```python
from build123d import *

# Parameters (mm, degrees)
F1_DEPTH = 20
F3_R     = 2
F5_DEPTH = 25
F6_R     = 2


with BuildPart() as f1:
    # F0 (on Front) → F1 (new body)
    with BuildSketch(Plane.XZ):
        with BuildLine():
            Line((-230, -180), (250, -180))
            ThreePointArc((250, -180), (264.142136, -174.142136), (270, -160))
            Line((270, -160), (270, -20))
            ThreePointArc((270, -20), (258.284271, 8.284271), (230, 20))
            Line((230, 20), (200, 20))
            Line((200, 20), (200, 140))
            ThreePointArc((200, 140), (188.284271, 168.284271), (160, 180))
            Line((160, 180), (-160, 180))
            ThreePointArc((-160, 180), (-188.284271, 168.284271), (-200, 140))
            Line((-200, 140), (-200, 20))
            Line((-200, 20), (-230, 20))
            ThreePointArc((-230, 20), (-258.284271, 8.284271), (-270, -20))
            Line((-270, -20), (-270, -140))
            ThreePointArc((-270, -140), (-258.284271, -168.284271), (-230, -180))
        make_face()
    extrude(amount=F1_DEPTH)

    # F3
    f3_edges = [f1.edges().sort_by_distance(p)[0] for p in [
        (10, -20, -180),
        (264.142136, -20, -174.142136),
        (270, -20, -90),
        (258.284271, -20, 8.284271),
        (215, -20, 20),
        (200, -20, 80),
        (188.284271, -20, 168.284271),
        (0, -20, 180),
        (-188.284271, -20, 168.284271),
        (-200, -20, 80),
        (-215, -20, 20),
        (-258.284271, -20, 8.284271),
        (-270, -20, -80),
        (-258.284271, -20, -168.284271),
        (10, 0, -180),
        (264.142136, 0, -174.142136),
        (270, 0, -90),
        (258.284271, 0, 8.284271),
        (215, 0, 20),
        (200, 0, 80),
        (188.284271, 0, 168.284271),
        (0, 0, 180),
        (-188.284271, 0, 168.284271),
        (-200, 0, 80),
        (-215, 0, 20),
        (-258.284271, 0, 8.284271),
        (-270, 0, -80),
        (-258.284271, 0, -168.284271),
    ]]
    fillet(f3_edges, radius=F3_R)

    # F4 (on face) → F5 (cut)
    with BuildSketch(Plane.XZ.offset(20)):
        with BuildLine():
            ThreePointArc((-14, -120), (10, -144), (34, -120))
            ThreePointArc((34, -120), (10, -96), (-14, -120))
        make_face()
    extrude(amount=-F5_DEPTH, mode=Mode.SUBTRACT)

    # F6
    f6_edges = [f1.edges().sort_by_distance(p)[0] for p in [
        (34, -20, -120),
        (34, 0, -120),
    ]]
    fillet(f6_edges, radius=F6_R)


solid = f1.part
```
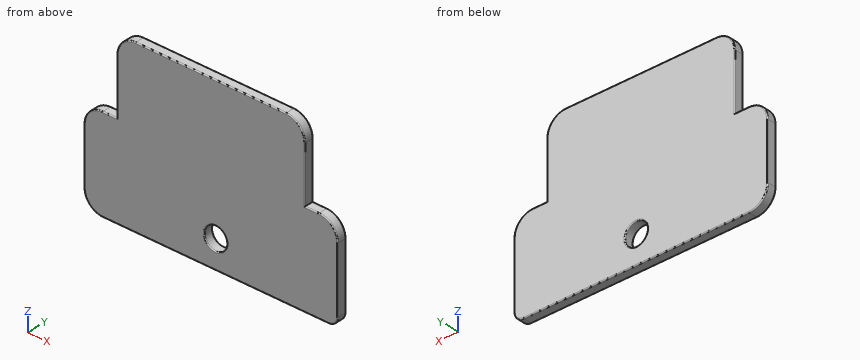
CAD build for the part. Positions are in the model's coordinates, mm. Coordinates: 2 decimals unless noted, no trailing zeros. Write each loop counter-clockwise with the first axis right and the second up, starting at its lowest first coordinate (ties: lowest second). Pieces come first, ordered by that corner, then holes.
(1) Cut at D-D, the plane z = 85. List the corners of the cut face in (x, y), and give its area (3 significant figures).
(2) Cut at A-A, the plane z = -120. List the corners of the cut face in (x, y), and give its area (3 significant figures).
(3) Flat gauge pins, fed straight in: pin 1 (8 mm diameter, centred on x = 210.5, y = -12, fed in from +Z); pin 2 (1 mm diameter, centred on y = -16, z = 100.5, fed in from -X); pin 3 (3 mm diameter, centred on x = -189.5, y = -12.5, fed in from +Z). Where does each tip first touch, or does it go through?
(4) Drill centre lines: probe 1 along Z at (x, y) = (10, -9); probe 2 along Z at (x, y) = (93.5, -18.25); probe 3 along Z at (x, y) = (217.5, -9.5). Where is each one in solid material? Low to high.
(5) Cut at C-C, the plane x = 10. List the corners of the cut face in (y, z).
(6) Cut at B-B, the plane y = -6. List the corners of the cut face in (x, z).
Geometry says:
1. outline: (-200, -18) arc R2 ccw to (-198, -20) - (198, -20) arc R2 ccw to (200, -18) - (200, -2) arc R2 ccw to (198, 0) - (-198, 0) arc R2 ccw to (-200, -2) - close
1. area: 8,000 mm2
2. outline: (-270, -18) arc R2 ccw to (-268, -20) - (-16, -20) arc R2 ccw to (-14, -18) - (-14, -2) arc R2 ccw to (-16, 0) - (-268, 0) arc R2 ccw to (-270, -2) - close; (34, -18) arc R2 ccw to (36, -20) - (268, -20) arc R2 ccw to (270, -18) - (270, -2) arc R2 ccw to (268, 0) - (36, 0) arc R2 ccw to (34, -2) - close
2. area: 9,830 mm2
3. pin 1: stops at z = 20
3. pin 2: stops at x = -200
3. pin 3: stops at z = 168.57
4. probe 1: z = -180 to -144, -96 to 180
4. probe 2: z = -179.98 to 179.98
4. probe 3: z = -180 to 20
5. outline: (-20, -178) arc R2 ccw to (-18, -180) - (-2, -180) arc R2 ccw to (0, -178) - (0, -146) arc R2 ccw to (-2, -144) - (-18, -144) arc R2 ccw to (-20, -146) - close; (-20, -94) arc R2 ccw to (-18, -96) - (-2, -96) arc R2 ccw to (0, -94) - (0, 178) arc R2 ccw to (-2, 180) - (-18, 180) arc R2 ccw to (-20, 178) - close
6. outline: (-270, -140) arc R40 ccw to (-230, -180) - (250, -180) arc R20 ccw to (270, -160) - (270, -20) arc R40 ccw to (230, 20) - (200, 20) - (200, 140) arc R40 ccw to (160, 180) - (-160, 180) arc R40 ccw to (-200, 140) - (-200, 20) - (-230, 20) arc R40 ccw to (-270, -20) - close; hole circle Ø48 at (10, -120)
